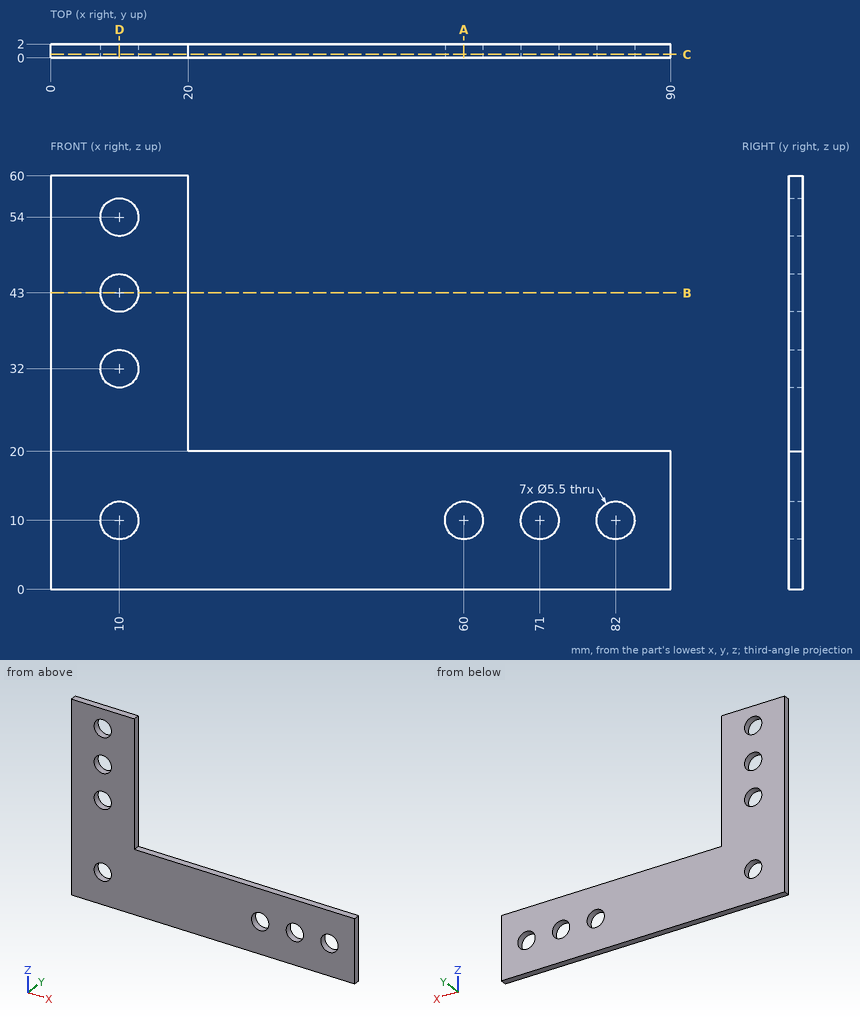
Answer from the drawing. Dimensions are ordinates in mm from the lowest x, y and z of the part. Coordinates: 2 decimals unless noted, no trailing zeros. Write each loop counter-clockwise with the first axis right and the second up, starting at its lowest first coordinate (ties: lowest second). Pieces come first, ordered by that corner, then holes. Notation, with made-up numbers: M 59.5,14.5 L 87.5,14.5 A15 ccw 87.5,37.5 Z; hole C 32,-22 d3. An arc over 180 degrees is marked long. Use a Markdown table: item, result.
Q1. The part is cut by section C-C, the plane y = 0.5. Write down the section's boundary in (x, z), then the cut area to 3 significant figures.
Answer block:
| item | result |
|---|---|
| outline | M 0,0 L 90,0 L 90,20 L 20,20 L 20,60 L 0,60 Z; hole C 10,10 d5.5; hole C 10,32 d5.5; hole C 10,43 d5.5; hole C 10,54 d5.5; hole C 60,10 d5.5; hole C 71,10 d5.5; hole C 82,10 d5.5 |
| area | 2,430 mm2 |
Q2. Straight lines are drawn through the part: L1, parallel to X at y = 1.45, z = 10; L2, parallel to Z at x = 26, y = 1.45; L3, parallel to X at y = 1.6, z = 54.5. For each, find the intervals that lie inside material, in ascending order. Write a range as [from, to].
Answer block:
| item | result |
|---|---|
| L1 | x = [0, 7.25], [12.75, 57.25], [62.75, 68.25], [73.75, 79.25], [84.75, 90] |
| L2 | z = [0, 20] |
| L3 | x = [0, 7.3], [12.7, 20] |
Q3. The part is cut by section D-D, the plane x = 10. Write down the section's boundary in (y, z).
Answer block:
| item | result |
|---|---|
| outline | M 0,0 L 2,0 L 2,7.25 L 0,7.25 Z; M 0,12.75 L 2,12.75 L 2,29.25 L 0,29.25 Z; M 0,34.75 L 2,34.75 L 2,40.25 L 0,40.25 Z; M 0,45.75 L 2,45.75 L 2,51.25 L 0,51.25 Z; M 0,56.75 L 2,56.75 L 2,60 L 0,60 Z |
Q4. The part is cut by section A-A, the plane x = 60. Write down the section's boundary in (y, z), then the cut area to 3 significant figures.
Answer block:
| item | result |
|---|---|
| outline | M 0,0 L 2,0 L 2,7.25 L 0,7.25 Z; M 0,12.75 L 2,12.75 L 2,20 L 0,20 Z |
| area | 29.0 mm2 |
Q5. The part is cut by section B-B, the plane z = 43. Write down the section's boundary in (x, y), then the cut area to 3 significant figures.
Answer block:
| item | result |
|---|---|
| outline | M 0,0 L 7.25,0 L 7.25,2 L 0,2 Z; M 12.75,0 L 20,0 L 20,2 L 12.75,2 Z |
| area | 29.0 mm2 |
Q6. This flat-tipped pin is pushed along its axis until it touches: pin 1 Ø0.6 at (x, y) = (45.5, 0.5) entering from +Z. Where does it stop, or does it pass through?
Answer block:
| item | result |
|---|---|
| pin 1 | stops at z = 20 |
